Answer from the drawing. Dimensions are ordinates in mm from the lowest x, y and z of the part. Give positions to 0.01 mm unless a question says otherwise; leave off trailing zeros. Write each loop counter-clockwise with the first axis right and the second up, starting at its lowest first coordinate (ties: lowest second). Pieces come first, ordered by that corner, then holes. Notation, with made-up numbers: (65.5, 0) -> (100.5, 0) arc R13 cw to (100.5, 5) -> close; hole circle Ø11 at (-38, 86). An arc over 180 degrees is marked (long way). Use a Markdown table: item, result. Add a question column.
Q1. Section B-B, the plane y = 239 is taken. Give the vertices of the cut face in (x, z) (1 decimal), plus the area to 3 significant figures.
Q2. This flat-tipped pin is pushed along its axis until it touches: pin 1 Ø15 at (y, z) = (15, 38) entering from +X. Where does it stop, or does it pass through?
Q3. Section C-C, the plane y = 285.5 is taken. Give the vertices of the cut face in (x, z) (1 decimal), plus the area to 3 significant figures.
Q4. Consider line 1 (X direction, y = 120.5, z = 25.5) (1 decimal); line 2 (Y direction, x = 240.5, z = 37.5); line 3 (Y direction, x = 101.5, z = 18). Determine where each line is inside the solid, lowest interval first.
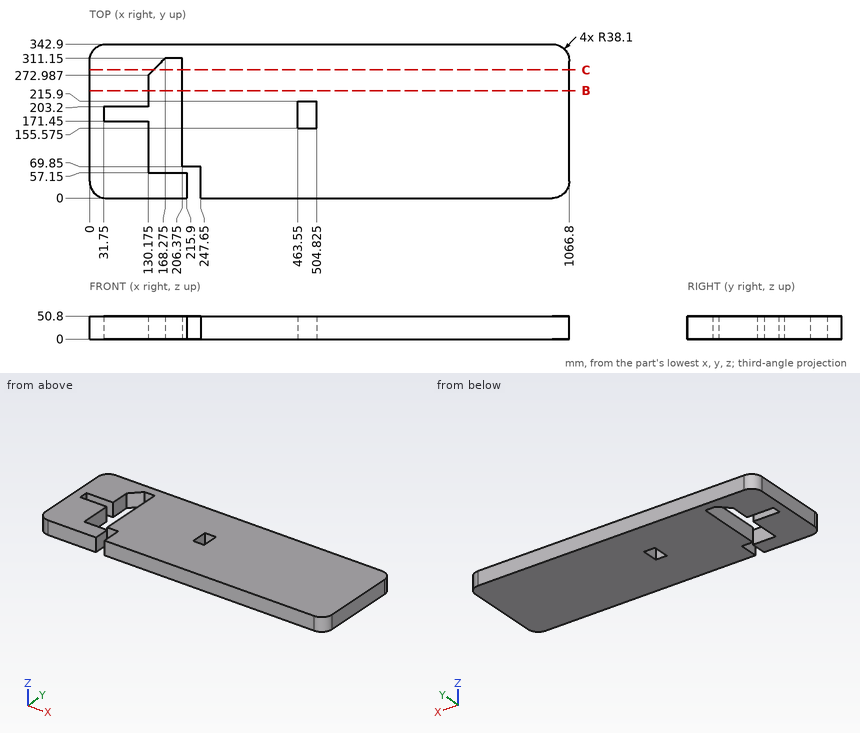
Result set:
| question | item | result |
|---|---|---|
| 1 | outline | (0, 0) -> (130.2, 0) -> (130.2, 50.8) -> (0, 50.8) -> close; (206.4, 0) -> (1066.8, 0) -> (1066.8, 50.8) -> (206.4, 50.8) -> close |
| 1 | area | 50,300 mm2 |
| 2 | pin 1 | stops at x = 1063.46 |
| 3 | outline | (0, 0) -> (142.7, 0) -> (142.7, 50.8) -> (0, 50.8) -> close; (206.4, 0) -> (1066.8, 0) -> (1066.8, 50.8) -> (206.4, 50.8) -> close |
| 3 | area | 51,000 mm2 |
| 4 | line 1 | x = 0 to 130.2, 206.4 to 1066.8 |
| 4 | line 2 | y = 69.85 to 342.9 |
| 4 | line 3 | y = 0 to 171.45, 203.2 to 342.9 |
